Read the model definition and answer for the solid it produces. Units are mm, in the model's axes. A direction names the side the tool comes from. Round coordinates to 2 decimals unless told otherwise and drop trailing zeros. Write each loop counter-clockwise with the first axis right and the second up, starting at its lowest first coordinate (ties: lowest second). Pieces come first, ordered by that corner, then holes.
from build123d import *

# Parameters (mm, degrees)
SKETCH1_R               = 12.5
BOSS_EXTRUDE1_DEPTH     = 20
SHELL1_START            = 4
SHELL1_DEPTH            = 12
CUT_EXTRUDE1_DEPTH      = 5
CUT_EXTRUDE2_DEPTH      = 48.668123521
CUT_EXTRUDE2_DEPTH_BACK = 48.668123521
SKETCH5_W               = 12.044517282
SKETCH5_H               = 4
SKETCH6_W               = 12
SKETCH6_H               = 4
BOSS_EXTRUDE2_DEPTH     = 20
SKETCH7_R               = 2
CUT_EXTRUDE3_DEPTH      = 51.062460986


# Read off the part's stored shape, not the designer's step: Shell1
with BuildPart() as part:
    # Sketch1 → Boss-Extrude1 (new body)
    with BuildSketch(Plane.XY):
        with BuildLine():
            Line((-2.738458484, 16.271166066), (-40, 10))
            Line((-40, 10), (-40, -10))
            Line((-40, -10), (-2.738458484, -16.271166066))
            ThreePointArc((-2.738458484, -16.271166066), (16.5, 0), (-2.738458484, 16.271166066))
        make_face()
        Circle(SKETCH1_R, mode=Mode.SUBTRACT)
    extrude(amount=BOSS_EXTRUDE1_DEPTH)

    # Shell1 outline → Shell1 (cut)
    with BuildSketch(Plane.XY.offset(SHELL1_START)):
        with BuildLine():
            Line((-36, -10.67320522), (-2.738458484, -16.271166065))
            ThreePointArc((-2.738458484, -16.271166065), (-15.467708297, -5.744562646), (-12.695548653, 10.539119716))
            Line((-12.695548653, 10.539119716), (-36, 6.616950141))
            Line((-36, 6.616950141), (-36, -10.67320522))
        make_face()
    extrude(amount=SHELL1_DEPTH, mode=Mode.SUBTRACT)

    # Sketch4 → Cut-Extrude1 (cut)
    with BuildSketch(Plane(origin=(-2.738458484, 16.271166066, 0), x_dir=(0.9861312767016037, 0.16596718082459888, 0), z_dir=(-0.16596718082459888, 0.9861312767016037, 0))):
        with BuildLine():
            Line((-23.80908583, -8.5), (-23.28557926, -8.5))
            Line((-23.28557926, -8.5), (-23.28557926, -11.5))
            Line((-23.28557926, -11.5), (-23.80908583, -11.5))
            ThreePointArc((-23.80908583, -11.5), (-27.78557926, -14.25), (-31.76207269, -11.5))
            Line((-31.76207269, -11.5), (-32.28557926, -11.5))
            Line((-32.28557926, -11.5), (-32.28557926, -8.5))
            Line((-32.28557926, -8.5), (-31.76207269, -8.5))
            ThreePointArc((-31.76207269, -8.5), (-27.78557926, -5.75), (-23.80908583, -8.5))
        make_face()
    extrude(amount=-CUT_EXTRUDE1_DEPTH, mode=Mode.SUBTRACT)

    # Sketch5 → Cut-Extrude2 (cut, two sides: drawn at the far end of the back side and taken through both)
    with BuildSketch(Plane.XY.offset(20).offset(-CUT_EXTRUDE2_DEPTH_BACK)):
        with Locations((16.5, 0)):
            Rectangle(SKETCH5_W, SKETCH5_H)
    extrude(amount=CUT_EXTRUDE2_DEPTH + CUT_EXTRUDE2_DEPTH_BACK, mode=Mode.SUBTRACT)

    # Sketch6 → Boss-Extrude2 (add)
    with BuildSketch(Plane.XY.offset(20)):
        with Locations((18.338962679, -4)):
            Rectangle(SKETCH6_W, SKETCH6_H)
        with Locations((18.338962679, 4)):
            Rectangle(SKETCH6_W, SKETCH6_H)
    extrude(amount=-BOSS_EXTRUDE2_DEPTH)

    # Sketch7 → Cut-Extrude3 (cut, through all)
    with BuildSketch(Plane(origin=(0, 6, 0), x_dir=(1, 0, 0), z_dir=(0, 1, 0))):
        with Locations(Location((19.854694414, -10, 0), (0, 0, 270))):
            Circle(SKETCH7_R)
    extrude(amount=-CUT_EXTRUDE3_DEPTH, mode=Mode.SUBTRACT)


solid = part.part
Q1. Section A-A (x = 0) is taken. Determine the outline of the cut face in (y, z).
Verdict:
outline: (-16.5, 0) - (-12.5, 0) - (-12.5, 20) - (-16.5, 20) - close; (12.5, 0) - (16.5, 0) - (16.5, 20) - (12.5, 20) - close
Q2. Section C-C (y = 0) is taken. Determine the outline of the cut face in (x, z), then the cut area to 3 significant figures.
Verdict:
outline: (-40, 0) - (-12.5, 0) - (-12.5, 20) - (-40, 20) - close; hole (-36, 4) - (-16.5, 4) - (-16.5, 16) - (-36, 16) - close
area: 316 mm2
Q3. Which of the six approach directions +Z, -Z, +X, -X, +Y, -Y give full straight-line access (tool end or side, diameter ignored) to faces 4 (the cylindrical face through (-29.88, 9.7, 5.75)), 5 (the flat face through (17, 2, 10)), 6 (the flat face through (-25.374, 10.462, 9.979))?
Verdict:
face 4: none
face 5: +Z, -Z, +X
face 6: -Y
Q4. Determine the mould class of faces 1 (the flat face through (-34, 9, 11.5)), 2 (the flat face through (-15, 0, 0)), 3 (the flat face through (24.339, -4, 10)) for opening direction Z: pulls with the +Z half, pulls with the -Z half, needs draft (parallel to the pull), parting line crosses it, or undercut.
Verdict:
face 1: undercut
face 2: pulls with the -Z half
face 3: needs draft
Q5. Straight lines are drawn through the part: probe 1 along Y at (x, z) = (-0.5, 14.5); probe 2 along Z at (x, y) = (-12, -13); probe 3 along X at (y, z) = (5, 5.25). For each, find the intervals that lie inside material, in ascending order.
Verdict:
probe 1: y = -16.49 to -12.49, 12.49 to 16.49
probe 2: z = 0 to 4, 16 to 20
probe 3: x = -40 to -36, -15.72 to -11.46, 11.46 to 24.34
Q6. Section D-D (z = 3) is taken. Determine the outline of the cut face in (x, y), then the cut area to 3 significant figures.
Verdict:
outline: (-40, -10) - (-2.74, -16.27) arc R16.5 ccw to (15.37, -6) - (24.34, -6) - (24.34, -2) - (12.34, -2) arc R12.5 cw (long way) to (12.34, 2) - (24.34, 2) - (24.34, 6) - (15.37, 6) arc R16.5 ccw to (-2.74, 16.27) - (-40, 10) - close
area: 1,060 mm2
Q7. Section B-B (z = 10) is taken. Determine the outline of the cut face in (x, y), then the cut area to 3 significant figures.
Verdict:
outline: (-40, -10) - (-36, -10.67) - (-36, 6.62) - (-33.91, 6.97) - (-34.58, 10.91) - (-40, 10) - close; (-25.7, 12.41) - (-25.04, 8.46) - (-12.7, 10.54) arc R16.5 ccw (long way) to (15.37, -6) - (17.85, -6) - (17.85, -2) - (12.34, -2) arc R12.5 cw (long way) to (12.34, 2) - (17.85, 2) - (17.85, 6) - (15.37, 6) arc R16.5 ccw to (-2.74, 16.27) - close; (21.85, -6) - (24.34, -6) - (24.34, -2) - (21.85, -2) - close; (21.85, 2) - (24.34, 2) - (24.34, 6) - (21.85, 6) - close
area: 537 mm2
Q8. Flat-ended cylindrical pins translate along their axes: pin 1 Ø10 at (x, z) = (19, 9) entering from -Y; pin 2 Ø8 at (x, z) = (-23.5, 11) entering from +Y; pin 3 Ø3 at (y, z) = (12, 7) entering from +X. Find the tip coordinate at first contact, or state that the pin passes through.
Verdict:
pin 1: stops at y = -8.73
pin 2: stops at y = 13.45
pin 3: stops at x = 12.73
